Input: dimensioned drawing with shaded views. Units: mm. Origin: part minimum x, y, z. Coordinates: 2 decimals unless noted, no trailing zeros. Loops run counter-clockwise (first coordinate to the right, second up) from the corner with the lowest first, then second, coordinate; pieces in that order, holes last.
Item 1: Section query C-C, the plane x = 26. Return the cut outline in (y, z).
Item 2: Section query B-B, the plane y = 43. Return the cut outline in (x, z), then the cut area to 3 significant figures.
Item 3: Section query A-A, the plane z = 2. Return the cut outline in (x, y).
Item 4: Line query: probe 1 along Y at (x, z) = (16, 1.25); probe 2 along X at (y, z) = (21, 6); probe 3 along Y at (x, z) = (144.5, 1.25). Output: solid intervals per line, ascending.
Item 5: Pin query (flat end, axial travel): pin 1 Ø3 at (x, z) = (8.5, 3) entering from -Y; pin 2 Ø3 at (y, z) = (2.5, 4) entering from -X; pin 3 Ø1.9 at (x, z) = (3.5, 4) entering from +Y. Return the tip coordinate at first contact, or that it passes through.
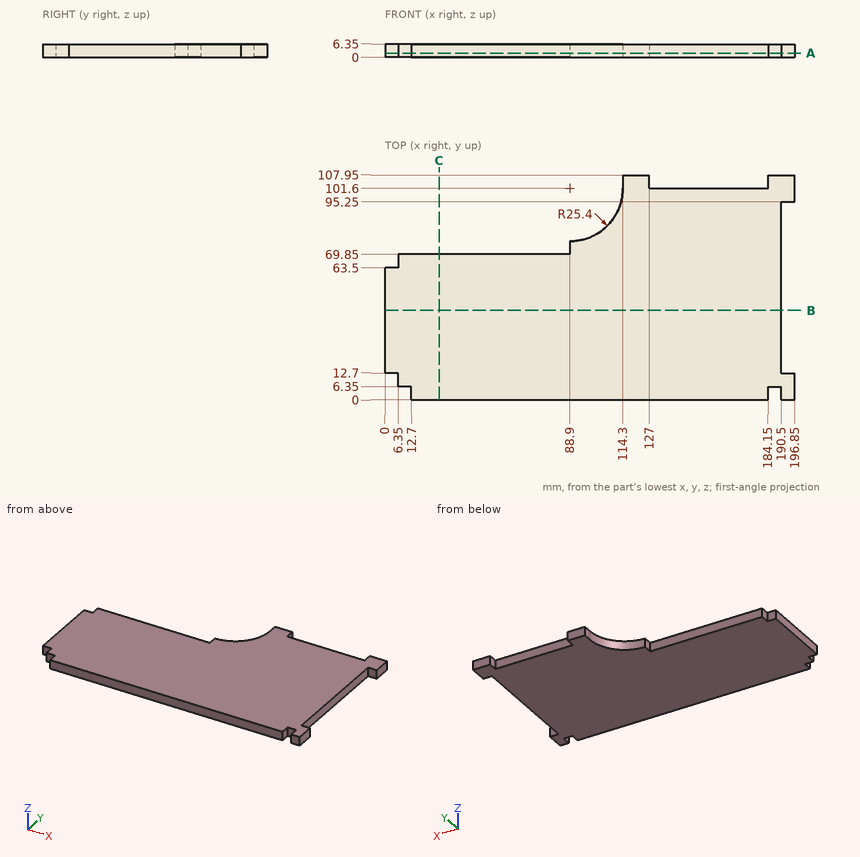
Verdict:
1. outline: (0, 0) - (69.85, 0) - (69.85, 6.35) - (0, 6.35) - close
2. outline: (0, 0) - (190.5, 0) - (190.5, 6.35) - (0, 6.35) - close
2. area: 1,210 mm2
3. outline: (0, 12.7) - (6.35, 12.7) - (6.35, 6.35) - (12.7, 6.35) - (12.7, 0) - (184.15, 0) - (184.15, 6.35) - (190.5, 6.35) - (190.5, 0) - (196.85, 0) - (196.85, 12.7) - (190.5, 12.7) - (190.5, 95.25) - (196.85, 95.25) - (196.85, 107.95) - (184.15, 107.95) - (184.15, 101.6) - (127, 101.6) - (127, 107.95) - (114.3, 107.95) - (114.3, 101.6) arc R25.4 cw to (88.9, 76.2) - (88.9, 69.85) - (6.35, 69.85) - (6.35, 63.5) - (0, 63.5) - close
4. probe 1: y = 0 to 69.85
4. probe 2: x = 0 to 190.5
4. probe 3: y = 0 to 101.6
5. pin 1: stops at y = 6.35
5. pin 2: stops at x = 12.7
5. pin 3: stops at y = 63.5
